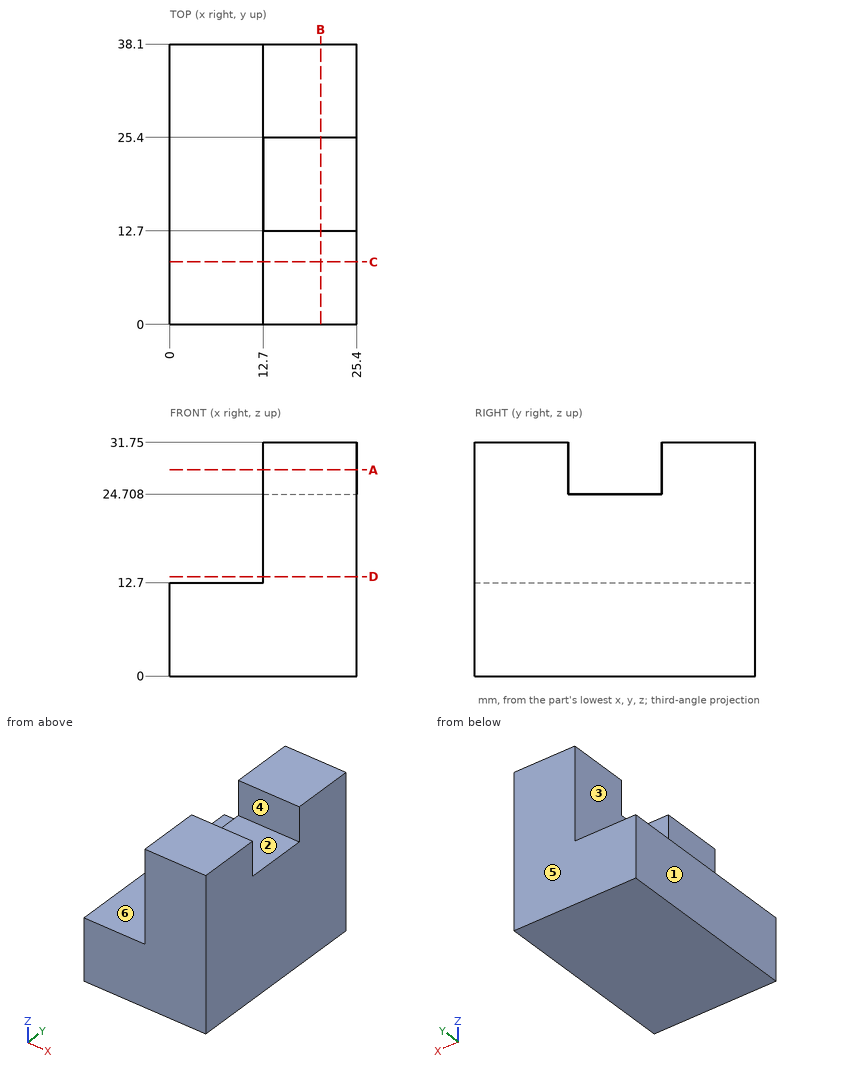
Source: three-view drawing plus pictorial views. Frame: mm from the lowest corner of the part. A direction names the side the tool comes from. Round coordinates to 2 decimals unless told otherwise and drop trailing zeros. Loops run counter-clockwise (first coordinate to the right, second up) from the corner with the lowest first, then second, coordinate; pieces in that order, holes last.
Q1. Pull-direction query (Y, two-part tool) for the marked faces 4, 5 and 6; classes: released by +Y, released by -Y, zero draft, split by the parting line, or undercut.
Q2. Pin query (flat end, axial travel): P1, Ø3, axis at y = 23, z = 18.5, coming from the -X side; P2, Ø8, axis at y = 16, z = 26, coming from the +X side; P3, Ø6.5, axis at x = 9, y = 12.5, coming from the +Z side; P4, Ø6.5, axis at x = 17, y = 20, coming from the +Z side. Return the tip coordinate at first contact, or that it passes through.
Q3. Section C-C on y = 8.5. Return loops of the section in (x, z).
Q4. Section B-B on x = 20.5. Return loops of the section in (y, z), plus the area to 3 significant figures.
Q5. Material intervals for L1, parallel to Y at x = 22.5, z = 27.5; L2, parallel to Z at x = 12.25, y = 9; L3, parallel to Z at x = 20.5, y = 16.5, sorted ascending.
Q6. Access query for the marked faces 1, 2 and 3. Directions: +Z, -Z, +X, -X, +Y, -Y. A direction counts if a zero-diameter tool reaches every point of the face in a straight line with its end or side. Return the directions, or none.
Q7. Section D-D on z = 13.5. Return loops of the section in (x, y).
Q8. Section A-A on z = 28. Return loops of the section in (x, y), plus the area to 3 significant figures.
Evaluation:
1. face 4: undercut
1. face 5: released by +Y
1. face 6: zero draft
2. P1: stops at x = 12.7
2. P2: stops at x = 25.4
2. P3: stops at z = 12.7
2. P4: stops at z = 24.71
3. outline: (0, 0) - (25.4, 0) - (25.4, 31.75) - (12.7, 31.75) - (12.7, 12.7) - (0, 12.7) - close
4. outline: (0, 0) - (38.1, 0) - (38.1, 31.75) - (25.4, 31.75) - (25.4, 24.71) - (12.7, 24.71) - (12.7, 31.75) - (0, 31.75) - close
4. area: 1,120 mm2
5. L1: y = 0 to 12.7, 25.4 to 38.1
5. L2: z = 0 to 12.7
5. L3: z = 0 to 24.71
6. face 1: +Z, -Z, -X, +Y, -Y
6. face 2: +Z, +X, -X
6. face 3: +Z, -X, +Y, -Y
7. outline: (12.7, 0) - (25.4, 0) - (25.4, 38.1) - (12.7, 38.1) - close
8. outline: (12.7, 0) - (25.4, 0) - (25.4, 12.7) - (12.7, 12.7) - close; (12.7, 25.4) - (25.4, 25.4) - (25.4, 38.1) - (12.7, 38.1) - close
8. area: 323 mm2
